Input: part model. Units: mm. Frame: model coordinates. Face numbers are marked on the shaded views. A direction names the side the tool comes from. Coordinates: 2 decimals unless noted, no trailing zeros. Loops run counter-clockwise (first coordinate to the right, second up) from the corner with the lowest first, then second, coordinate; pieces in that order, holes last.
(1) Section C-C, the plane y = -11. Return loops of the section in (x, z), then the cut area to 3 significant figures.
(2) Section A-A, the plane z = 0. Return loops of the section in (x, y).
(3) Line query: L1, parallel to Z at x = -19, y = 0; L2, parallel to Z at x = -20.5, y = -21.5; L3, parallel to X at y = 15, z = -38. Output: solid intervals per line, ascending.
(4) Section D-D, the plane z = -41.5. Return loops of the section in (x, y).
(5) Section B-B, the plane x = 11.5. Return loops of the section in (y, z), then the cut area to 3 significant figures.
(6) Contact query for flat-ended pins moving along their axis: P1, Ø8, axis at y = -4, z = -51, coming from the -X side; P2, Ø1.5, axis at y = 0, z = 1, coming from the -X side. Output: stop coordinate, or through.
(7) Set-up query: the marked faces 1, 2, 3, 4 and 5. Return all of +Z, -Z, +X, -X, +Y, -Y with unobstructed straight access to the full face (end or side cutting, diameter ignored); none if empty.
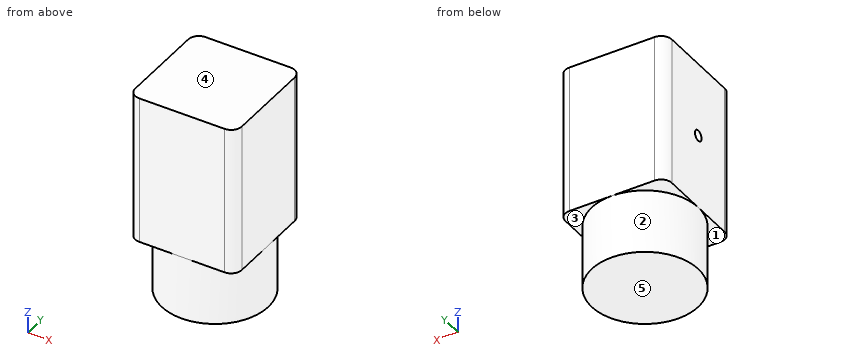
```python
from build123d import *

# Parameters (mm, degrees)
F0_W     = 50
F0_H     = 70
F1_DEPTH = 25
F2_R     = 25
F3_DEPTH = 30
F4_R     = 5
F5_R     = 2.5
F6_DEPTH = 10


with BuildPart() as f1:
    # F0 (on Front) → F1 (new body, symmetric)
    with BuildSketch(Plane.XZ):
        Rectangle(F0_W, F0_H)
    extrude(amount=F1_DEPTH, both=True)

    # F2 (on face) → F3 (join)
    with BuildSketch(Plane(origin=(0, 0, -35), x_dir=(1, 0, 0), z_dir=(0, 0, -1))):
        Circle(F2_R)
    extrude(amount=F3_DEPTH)

    # F4
    f4_edges = [f1.edges().sort_by_distance(p)[0] for p in [
        (25, -25, 0),
        (-25, -25, 0),
        (-25, 25, 0),
        (25, 25, 0),
    ]]
    fillet(f4_edges, radius=F4_R)

    # F5 (on face) → F6 (cut)
    with BuildSketch(Plane(origin=(-25, 0, 0), x_dir=(0, -1, 0), z_dir=(-1, 0, 0))):
        Circle(F5_R)
    extrude(amount=-F6_DEPTH, mode=Mode.SUBTRACT)


solid = f1.part
```
Report:
1. outline: (-25, -35) - (-22.45, -35) - (-22.45, -65) - (22.45, -65) - (22.45, -35) - (25, -35) - (25, 35) - (-25, 35) - close
1. area: 4,850 mm2
2. outline: (-25, -20) arc R5 ccw to (-20, -25) - (20, -25) arc R5 ccw to (25, -20) - (25, 20) arc R5 ccw to (20, 25) - (-20, 25) arc R5 ccw to (-25, 20) - (-25, 2.5) - (-15, 2.5) - (-15, -2.5) - (-25, -2.5) - close
3. L1: z = -65 to -2.5, 2.5 to 35
3. L2: z = -35 to 35
3. L3: x = -20 to 20
4. outline: circle Ø50 at (0, 0)
5. outline: (-25, -35) - (-22.2, -35) - (-22.2, -65) - (22.2, -65) - (22.2, -35) - (25, -35) - (25, 35) - (-25, 35) - close
5. area: 4,830 mm2
6. P1: stops at x = -25
6. P2: stops at x = -15
7. face 1: -Z, -X, -Y
7. face 2: -Z
7. face 3: -Z, +X, +Y
7. face 4: +Z, +X, -X, +Y, -Y
7. face 5: -Z, +X, -X, +Y, -Y
